Verification items for the finished model (mm, model axes). Face numbers are marked on the shaded views. A direction names the side the tool comes from. Coordinates: 2 decimals unless noted, no trailing zeros. Loops run counter-clockwise (first coordinate to the right, second up) from the corner with the lowest first, then second, coordinate; pieces in that order, holes last.
Q1. Sectioned sample at D-D (x = 16.5). Enter the section's corners in (y, z) (3 decimals).
Q2. Mould release check, pull along X, two halves, no side actions. Record for the marked faces 4, 5, 6 and 7: +X half, -X half, draft (parallel to the pull), parting line (faces both ways), or undercut.
Q3. Sectioned sample at B-B (z = -8.5). Enter the section's corners in (x, y) (3 decimals), then the cut area to 3 significant figures.
Q4. Sectioned sample at A-A (y = 0.8). Enter the section's corners in (x, z) (3 decimals).
Q5. Access from +Z, -Z, +X, -X, +Y, -Y to the whole of each face (thin tool, end or side, straight path). Record for the marked faces 1, 2 and 3.
Q6. Sectioned sample at C-C (z = 4.5). Enter the section's corners in (x, y) (1 decimal).
Q7. Go/stop test with flat-tipped pins: P1, Ø1, axis at y = 2, z = -15.5, coming from the -X side; P2, Ø1, axis at x = 15.5, y = 1, coming from the +Z side. Record where each tip stops, or that it passes through.
Q8. Material ranges on probe 1 along X at (y, z) = (1.9, 0); probe 2 along Z at (x, y) = (0, 1.8) (3 decimals); probe 3 along X at (y, z) = (1.7, -4.5), recorded low to high.
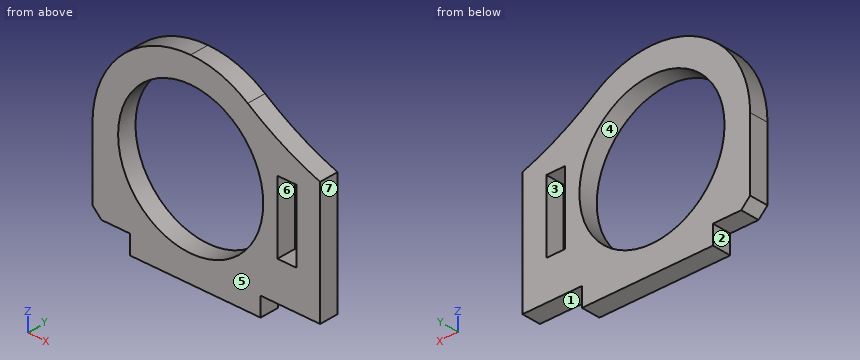
```python
from build123d import *

# Parameters (mm, degrees)
BOSS_EXTRUDE1_DEPTH = 3.175
SKETCH2_W           = 3.175
SKETCH2_H           = 14
BOSS_EXTRUDE2_DEPTH = 3.175
BOSS_EXTRUDE3_DEPTH = 3.175
CUT_EXTRUDE2_START  = -10
CUT_EXTRUDE2_DEPTH  = 10
FILLET1_R           = 50
SKETCH6_W           = 6.875
SKETCH6_H           = 3.175
BOSS_EXTRUDE5_DEPTH = 3.11351312
SKETCH7_W           = 11.175
SKETCH7_H           = 3.175
SKETCH7_W_2         = 4.3
CUT_EXTRUDE3_DEPTH  = 5.11351312
BOSS_EXTRUDE6_START = -3.175
BOSS_EXTRUDE6_DEPTH = 3.175
SKETCH9_W           = 3.175
SKETCH9_H           = 14
BOSS_EXTRUDE7_DEPTH = 3.175
SKETCH10_W          = 3.175
SKETCH10_H          = 12
CUT_EXTRUDE4_DEPTH  = 3.175
CUT_EXTRUDE5_DEPTH  = 10
SKETCH14_W          = 22
SKETCH14_H          = 3.175
BOSS_EXTRUDE8_DEPTH = 3.175
CHAMFER1_SIZE       = 1.5


with BuildPart() as part:
    # Sketch1 → Boss-Extrude1 (new body)
    with BuildSketch(Plane(origin=(0, 0, 0), x_dir=(1, 0, 0), z_dir=(0, 1, 0))):
        with BuildLine():
            ThreePointArc((-16.5, 0), (0, -16.5), (16.5, 0))
            Line((16.5, 0), (16.5, 18.61351312))
            Line((16.5, 18.61351312), (12.2, 18.61351312))
            Line((12.2, 18.61351312), (12.2, 0))
            ThreePointArc((12.2, 0), (0, -12.2), (-12.2, 0))
            Line((-12.2, 0), (-12.2, 18))
            Line((-12.2, 18), (-16.5, 18))
            Line((-16.5, 18), (-16.5, 0))
        make_face()
    extrude(amount=BOSS_EXTRUDE1_DEPTH)

    # Sketch2 → Boss-Extrude2 (add)
    with BuildSketch(Plane(origin=(0, 3.175, 0), x_dir=(1, 0, 0), z_dir=(0, 1, 0))):
        with BuildLine():
            Line((15.2, -3.034798181), (15.2, -4.5))
            Line((15.2, -4.5), (15.874507866, -4.5))
            Line((15.874507866, -4.5), (23.375, -4.5))
            Line((23.375, -4.5), (23.375, 15.5))
            Line((23.375, 15.5), (15.2, 15.5))
            Line((15.2, 15.5), (15.2, 3.034798181))
            ThreePointArc((15.2, 3.034798181), (15.424817665, 1.524795068), (15.5, 0))
            ThreePointArc((15.5, 0), (15.424817665, -1.524795068), (15.2, -3.034798181))
        make_face()
        with Locations((18.0875, 4.5)):
            Rectangle(SKETCH2_W, SKETCH2_H, mode=Mode.SUBTRACT)
    extrude(amount=-BOSS_EXTRUDE2_DEPTH)

    # Sketch3 → Boss-Extrude3 (add)
    with BuildSketch(Plane(origin=(0, 0, 0), x_dir=(-1, 0, 0), z_dir=(0, -1, 0))):
        with BuildLine():
            Line((-23.375, -16.5), (0, -16.5))
            ThreePointArc((0, -16.5), (-9.949874371, -13.162446581), (-15.874507866, -4.5))
            Line((-15.874507866, -4.5), (-23.375, -4.5))
            Line((-23.375, -4.5), (-23.375, -16.5))
        make_face()
    extrude(amount=-BOSS_EXTRUDE3_DEPTH)

    # Sketch5 → Cut-Extrude2 (cut)
    with BuildSketch(Plane(origin=(0, 3.175, 0), x_dir=(1, 0, 0), z_dir=(0, 1, 0)).offset(CUT_EXTRUDE2_START)):
        with BuildLine():
            Line((23.375, -6.5), (19.675, -6.5))
            Line((19.675, -6.5), (17.491400843, -6.5))
            Line((17.491400843, -6.5), (15.165750888, -6.5))
            ThreePointArc((15.165750888, -6.5), (9.082951062, -13.774977314), (0, -16.5))
            Line((0, -16.5), (12.165525061, -16.5))
            Line((12.165525061, -16.5), (23.375, -16.5))
            Line((23.375, -16.5), (23.375, -6.5))
        make_face()
    extrude(amount=CUT_EXTRUDE2_DEPTH, mode=Mode.SUBTRACT)

    # Fillet1
    # the kernel refuses this fillet: 50 mm, written as the material it adds along each edge
    with BuildSketch(Plane(origin=(15.165750888, 0, 6.5), x_dir=(-0.6269455789999085, 0, 0.7790630532713443), z_dir=(0, 1, 0))) as fillet1_piece_1:
        with BuildLine():
            CenterArc((22.355625569, 48.152189259), FILLET1_R, 236.629724146, 17.744988352)
            Line((-5.146752438, 6.395522678), (-5.696799998, 5.560389347))
            ThreePointArc((-5.696799998, 5.560389347), (-3.352439272, 2.57081576), (-0.779063053, -0.626945579))
            Line((-0.779063053, -0.626945579), (0.269344886, -0.963043785))
            ThreePointArc((0.269344886, -0.963043785), (4.444190625, -0.390222456), (8.619036364, -0.963043785))
            Line((8.619036364, -0.963043785), (8.88838125, 0))
        make_face()
    extrude(amount=3.175)

    # Sketch6 → Boss-Extrude5 (add)
    with BuildSketch(Plane(origin=(0, 0, -15.5), x_dir=(-1, 0, 0), z_dir=(0, 0, -1))):
        with Locations((-19.9375, 1.5875)):
            Rectangle(SKETCH6_W, SKETCH6_H)
    extrude(amount=BOSS_EXTRUDE5_DEPTH)

    # Sketch7 → Cut-Extrude3 (cut)
    with BuildSketch(Plane(origin=(0, 0, -18.61351312), x_dir=(-1, 0, 0), z_dir=(0, 0, -1))):
        with Locations((-17.7875, 1.5875)):
            Rectangle(SKETCH7_W, SKETCH7_H)
        with Locations((14.35, 1.5875)):
            Rectangle(SKETCH7_W_2, SKETCH7_H)
    extrude(amount=-CUT_EXTRUDE3_DEPTH, mode=Mode.SUBTRACT)

    # Sketch8 → Boss-Extrude6 (add)
    with BuildSketch(Plane(origin=(0, 3.175, 0), x_dir=(1, 0, 0), z_dir=(0, 1, 0)).offset(BOSS_EXTRUDE6_START)):
        with BuildLine():
            Line((-12.2, 13.5), (-12.2, 0))
            ThreePointArc((-12.2, 0), (0, 12.2), (12.2, 0))
            Line((12.2, 0), (12.2, 13.5))
            Line((12.2, 13.5), (-12.2, 13.5))
        make_face()
    extrude(amount=BOSS_EXTRUDE6_DEPTH)

    # Sketch9 → Boss-Extrude7 (add)
    with BuildSketch(Plane(origin=(0, 0, 0), x_dir=(-1, 0, 0), z_dir=(0, -1, 0))):
        with Locations((-18.0875, 4.5)):
            Rectangle(SKETCH9_W, SKETCH9_H)
    extrude(amount=-BOSS_EXTRUDE7_DEPTH)

    # Sketch10 → Cut-Extrude4 (cut)
    with BuildSketch(Plane(origin=(0, 0, 0), x_dir=(-1, 0, 0), z_dir=(0, -1, 0))):
        with Locations((-16.17406463, 1)):
            Rectangle(SKETCH10_W, SKETCH10_H)
    extrude(amount=-CUT_EXTRUDE4_DEPTH, mode=Mode.SUBTRACT)

    # Sketch12 → Cut-Extrude5 (cut)
    with BuildSketch(Plane(origin=(0, 0, 0), x_dir=(-1, 0, 0), z_dir=(0, -1, 0))):
        with BuildLine():
            Line((-21.76156463, -7.048663108), (-21.76156463, 13.5))
            Line((-21.76156463, 13.5), (-23.375, 13.5))
            Line((-23.375, 13.5), (-23.375, -6.5))
            ThreePointArc((-23.375, -6.5), (-22.565944603, -6.767457123), (-21.76156463, -7.048663108))
        make_face()
    extrude(amount=-CUT_EXTRUDE5_DEPTH, mode=Mode.SUBTRACT)

    # Sketch14 → Boss-Extrude8 (add)
    with BuildSketch(Plane(origin=(0, 0, -13.5), x_dir=(-1, 0, 0), z_dir=(0, 0, -1))):
        with Locations((-0.76156463, 1.5875)):
            Rectangle(SKETCH14_W, SKETCH14_H)
    extrude(amount=BOSS_EXTRUDE8_DEPTH)

    # Chamfer1
    chamfer1_edges = [part.edges().sort_by_distance(p)[0] for p in [
        (-16.5, 1.5875, -13.5),
    ]]
    chamfer(chamfer1_edges, length=CHAMFER1_SIZE)


solid = part.part
```
Geometry check:
1. outline: (0, -13.5) - (3.175, -13.5) - (3.175, -7) - (0, -7) - close; (0, 5) - (3.175, 5) - (3.175, 9.286) - (0, 9.286) - close
2. face 4: undercut
2. face 5: draft
2. face 6: undercut
2. face 7: +X half
3. outline: (-16.5, 0) - (-8.752, 0) - (-8.752, 3.175) - (-16.5, 3.175) - close; (8.752, 0) - (21.762, 0) - (21.762, 3.175) - (8.752, 3.175) - close
3. area: 65.9 mm2
4. outline: (-16.5, -12) - (-15, -13.5) - (-10.238, -13.5) - (-10.238, -16.675) - (11.762, -16.675) - (11.762, -13.5) - (21.762, -13.5) - (21.762, 7.049) arc R50 cw to (9.593, 13.425) arc R16.5 ccw to (-16.5, 0) - close; hole circle Ø24.4 at (0, 0); hole (14.587, -7) - (17.762, -7) - (17.762, 5) - (14.587, 5) - close
5. face 1: -Z, +X, +Y, -Y
5. face 2: -Z, -X, +Y, -Y
5. face 3: +Y, -Y
6. outline: (-15.9, 0) - (-11.3, 0) - (-11.3, 3.2) - (-15.9, 3.2) - close; (11.3, 0) - (14.6, 0) - (14.6, 3.2) - (11.3, 3.2) - close; (17.8, 0) - (21.8, 0) - (21.8, 3.2) - (17.8, 3.2) - close
7. P1: stops at x = -10.24
7. P2: stops at z = 10.06
8. probe 1: x = -16.5 to -12.2, 12.2 to 14.59, 17.76 to 21.76
8. probe 2: z = -16.675 to -12.2, 12.2 to 16.5
8. probe 3: x = -16.5 to -11.34, 11.34 to 14.59, 17.76 to 21.76
